Source: CAD feature listing. Evaluate the final solid. Frame: model axes, mm. Give positions to 0.01 mm unless a question says otherwise; leave off trailing zeros. Write each loop counter-clockwise with the first axis right and the second up, starting at its lowest first coordinate (ties: lowest second). Pieces come first, ordered by that corner, then holes. Notation, with made-up numbers: (23, -0.5) -> (47, -0.5) arc R34 ccw to (47, 33.5) -> close; hole circle Ø1 at (-11.5, 67). An arc over 180 degrees is marked (long way). Use a Markdown table: item, result. Add a question column.
```python
from build123d import *

# Parameters (mm, degrees)
BOSS_EXTRUDE1_DEPTH = 6
SKETCH2_R           = 12.45
BOSS_EXTRUDE2_DEPTH = 5.25
CUT_EXTRUDE2_REACH  = 13.25
SKETCH5_R           = 1.6
SKETCH6_R           = 2.75
CUT_EXTRUDE3_DEPTH  = 3.2
SKETCH7_R           = 2.75
CUT_EXTRUDE4_DEPTH  = 3.2
CUT_EXTRUDE7_REACH  = 8
SKETCH10_R          = 9.95
CUT_EXTRUDE8_REACH  = 13.25
SKETCH11_R          = 1.6
SKETCH12_R          = 2.75
CUT_EXTRUDE9_DEPTH  = 3
CUT_EXTRUDE10_DEPTH = 3
CUT_EXTRUDE11_REACH = 13.25
SKETCH14_R          = 1.6
SKETCH15_R          = 2.75
CUT_EXTRUDE12_DEPTH = 1.5
CUT_EXTRUDE13_REACH = 13.25
SKETCH16_R          = 1.1


with BuildPart() as part:
    # Sketch1 → Boss-Extrude1 (new body)
    with BuildSketch(Plane.XY):
        with BuildLine():
            Line((53.452478751, 19.630204959), (350.418509131, 15.138345609))
            ThreePointArc((350.418509131, 15.138345609), (370.113739503, -5.161848985), (349.813544909, -24.857079358))
            Line((349.813544909, -24.857079358), (52.847514529, -20.365220008))
            ThreePointArc((52.847514529, -20.365220008), (33.152284157, -0.065025413), (53.452478751, 19.630204959))
        make_face()
    extrude(amount=BOSS_EXTRUDE1_DEPTH)

    # Sketch2 → Boss-Extrude2 (add)
    with BuildSketch(Plane(origin=(0, 0, 0), x_dir=(-1, 0, 0), z_dir=(0, 0, -1))):
        with Locations((-53.14999664, -0.367507524)):
            Circle(SKETCH2_R)
    extrude(amount=BOSS_EXTRUDE2_DEPTH)

    # Sketch5 → Cut-Extrude2 (cut, up to next)
    with BuildSketch(Plane.XY.offset(6), mode=Mode.PRIVATE) as cut_extrude2_sk1:
        with Locations((80.82937417, 15.215648985)):
            Circle(SKETCH5_R)
    cut_extrude2_tool1 = extrude(cut_extrude2_sk1.sketch, amount=-CUT_EXTRUDE2_REACH, mode=Mode.PRIVATE) & part.part
    add(cut_extrude2_tool1.solids().sort_by_distance((80.829374, 15.215649, 6))[0], mode=Mode.SUBTRACT)
    # Sketch5 → Cut-Extrude2 (cut, up to next)
    with BuildSketch(Plane.XY.offset(6), mode=Mode.PRIVATE) as cut_extrude2_sk2:
        with Locations((46.471460884, -0.26648909)):
            Circle(SKETCH5_R)
    cut_extrude2_tool2 = extrude(cut_extrude2_sk2.sketch, amount=-CUT_EXTRUDE2_REACH, mode=Mode.PRIVATE) & part.part
    add(cut_extrude2_tool2.solids().sort_by_distance((46.471461, -0.266489, 6))[0], mode=Mode.SUBTRACT)
    # Sketch5 → Cut-Extrude2 (cut, up to next)
    with BuildSketch(Plane.XY.offset(6), mode=Mode.PRIVATE) as cut_extrude2_sk3:
        with Locations((80.345467382, -16.77642084)):
            Circle(SKETCH5_R)
    cut_extrude2_tool3 = extrude(cut_extrude2_sk3.sketch, amount=-CUT_EXTRUDE2_REACH, mode=Mode.PRIVATE) & part.part
    add(cut_extrude2_tool3.solids().sort_by_distance((80.345467, -16.776421, 6))[0], mode=Mode.SUBTRACT)

    # Sketch6 → Cut-Extrude3 (cut)
    with BuildSketch(Plane(origin=(0, 0, 0), x_dir=(-1, 0, 0), z_dir=(0, 0, -1))):
        with Locations((-80.345467382, -16.77642084)):
            Circle(SKETCH6_R)
        with Locations((-80.82937417, 15.215648985)):
            Circle(SKETCH6_R)
    extrude(amount=-CUT_EXTRUDE3_DEPTH, mode=Mode.SUBTRACT)

    # Sketch7 → Cut-Extrude4 (cut)
    with BuildSketch(Plane(origin=(0, 0, -5.25), x_dir=(-1, 0, 0), z_dir=(0, 0, -1))):
        with Locations((-46.471460884, -0.26648909)):
            Circle(SKETCH7_R)
    extrude(amount=-CUT_EXTRUDE4_DEPTH, mode=Mode.SUBTRACT)

    # Sketch10 → Cut-Extrude7 (cut, up to next)
    with BuildSketch(Plane(origin=(0, 0, 0), x_dir=(-1, 0, 0), z_dir=(0, 0, -1)), mode=Mode.PRIVATE) as cut_extrude7_sk1:
        with Locations((-350.11602702, -4.859366874)):
            Circle(SKETCH10_R)
    cut_extrude7_tool1 = extrude(cut_extrude7_sk1.sketch, amount=-CUT_EXTRUDE7_REACH, mode=Mode.PRIVATE) & part.part
    add(cut_extrude7_tool1.solids().sort_by_distance((350.116027, -4.859367, 0))[0], mode=Mode.SUBTRACT)

    # Sketch11 → Cut-Extrude8 (cut, up to next)
    with BuildSketch(Plane.XY.offset(6), mode=Mode.PRIVATE) as cut_extrude8_sk1:
        with Locations((207.693855596, 5.295802586)):
            Circle(SKETCH11_R)
    cut_extrude8_tool1 = extrude(cut_extrude8_sk1.sketch, amount=-CUT_EXTRUDE8_REACH, mode=Mode.PRIVATE) & part.part
    add(cut_extrude8_tool1.solids().sort_by_distance((207.693856, 5.295803, 6))[0], mode=Mode.SUBTRACT)
    # Sketch11 → Cut-Extrude8 (cut, up to next)
    with BuildSketch(Plane.XY.offset(6), mode=Mode.PRIVATE) as cut_extrude8_sk2:
        with Locations((207.451869907, -10.702367401)):
            Circle(SKETCH11_R)
    cut_extrude8_tool2 = extrude(cut_extrude8_sk2.sketch, amount=-CUT_EXTRUDE8_REACH, mode=Mode.PRIVATE) & part.part
    add(cut_extrude8_tool2.solids().sort_by_distance((207.45187, -10.702367, 6))[0], mode=Mode.SUBTRACT)
    # Sketch11 → Cut-Extrude8 (cut, up to next)
    with BuildSketch(Plane.XY.offset(6), mode=Mode.PRIVATE) as cut_extrude8_sk3:
        with Locations((168.025770935, 5.895815512)):
            Circle(SKETCH11_R)
    cut_extrude8_tool3 = extrude(cut_extrude8_sk3.sketch, amount=-CUT_EXTRUDE8_REACH, mode=Mode.PRIVATE) & part.part
    add(cut_extrude8_tool3.solids().sort_by_distance((168.025771, 5.895816, 6))[0], mode=Mode.SUBTRACT)
    # Sketch11 → Cut-Extrude8 (cut, up to next)
    with BuildSketch(Plane.XY.offset(6), mode=Mode.PRIVATE) as cut_extrude8_sk4:
        with Locations((167.783785246, -10.102354474)):
            Circle(SKETCH11_R)
    cut_extrude8_tool4 = extrude(cut_extrude8_sk4.sketch, amount=-CUT_EXTRUDE8_REACH, mode=Mode.PRIVATE) & part.part
    add(cut_extrude8_tool4.solids().sort_by_distance((167.783785, -10.102354, 6))[0], mode=Mode.SUBTRACT)

    # Sketch12 → Cut-Extrude9 (cut)
    with BuildSketch(Plane(origin=(0, 0, 0), x_dir=(-1, 0, 0), z_dir=(0, 0, -1))):
        with Locations((-207.451869907, -10.702367401)):
            Circle(SKETCH12_R)
        with Locations((-207.693855596, 5.295802586)):
            Circle(SKETCH12_R)
        with Locations((-168.025770935, 5.895815512)):
            Circle(SKETCH12_R)
        with Locations((-167.783785246, -10.102354474)):
            Circle(SKETCH12_R)
    extrude(amount=-CUT_EXTRUDE9_DEPTH, mode=Mode.SUBTRACT)

    # Sketch13 → Cut-Extrude10 (cut)
    with BuildSketch(Plane.XY.offset(6)):
        Polygon((289.732546516, 16.056271502), (289.422502353, -4.441383793), (320.418956702, -4.910231066), (320.729000866, 15.58742423), align=None)
    extrude(amount=-CUT_EXTRUDE10_DEPTH, mode=Mode.SUBTRACT)

    # Sketch14 → Cut-Extrude11 (cut, up to next)
    with BuildSketch(Plane.XY.offset(6), mode=Mode.PRIVATE) as cut_extrude11_sk1:
        with Locations((312.048483794, 3.717351637)):
            Circle(SKETCH14_R)
    cut_extrude11_tool1 = extrude(cut_extrude11_sk1.sketch, amount=-CUT_EXTRUDE11_REACH, mode=Mode.PRIVATE) & part.part
    add(cut_extrude11_tool1.solids().sort_by_distance((312.048484, 3.717352, 6))[0], mode=Mode.SUBTRACT)
    # Sketch14 → Cut-Extrude11 (cut, up to next)
    with BuildSketch(Plane.XY.offset(6), mode=Mode.PRIVATE) as cut_extrude11_sk2:
        with Locations((298.050085055, 3.929089115)):
            Circle(SKETCH14_R)
    cut_extrude11_tool2 = extrude(cut_extrude11_sk2.sketch, amount=-CUT_EXTRUDE11_REACH, mode=Mode.PRIVATE) & part.part
    add(cut_extrude11_tool2.solids().sort_by_distance((298.050085, 3.929089, 6))[0], mode=Mode.SUBTRACT)

    # Sketch15 → Cut-Extrude12 (cut)
    with BuildSketch(Plane(origin=(0, 0, 0), x_dir=(-1, 0, 0), z_dir=(0, 0, -1))):
        with Locations((-298.050085055, 3.929089115)):
            Circle(SKETCH15_R)
        with Locations((-312.048483794, 3.717351637)):
            Circle(SKETCH15_R)
    extrude(amount=-CUT_EXTRUDE12_DEPTH, mode=Mode.SUBTRACT)

    # Sketch16 → Cut-Extrude13 (cut, up to next)
    with BuildSketch(Plane.XY.offset(6), mode=Mode.PRIVATE) as cut_extrude13_sk1:
        with Locations((92.548117071, 17.038621984)):
            Circle(SKETCH16_R)
    cut_extrude13_tool1 = extrude(cut_extrude13_sk1.sketch, amount=-CUT_EXTRUDE13_REACH, mode=Mode.PRIVATE) & part.part
    add(cut_extrude13_tool1.solids().sort_by_distance((92.548117, 17.038622, 6))[0], mode=Mode.SUBTRACT)
    # Sketch16 → Cut-Extrude13 (cut, up to next)
    with BuildSketch(Plane.XY.offset(6), mode=Mode.PRIVATE) as cut_extrude13_sk2:
        with Locations((92.003649271, -18.957260486)):
            Circle(SKETCH16_R)
    cut_extrude13_tool2 = extrude(cut_extrude13_sk2.sketch, amount=-CUT_EXTRUDE13_REACH, mode=Mode.PRIVATE) & part.part
    add(cut_extrude13_tool2.solids().sort_by_distance((92.003649, -18.95726, 6))[0], mode=Mode.SUBTRACT)
    # Sketch16 → Cut-Extrude13 (cut, up to next)
    with BuildSketch(Plane.XY.offset(6), mode=Mode.PRIVATE) as cut_extrude13_sk3:
        with Locations((151.905473082, 16.140792376)):
            Circle(SKETCH16_R)
    cut_extrude13_tool3 = extrude(cut_extrude13_sk3.sketch, amount=-CUT_EXTRUDE13_REACH, mode=Mode.PRIVATE) & part.part
    add(cut_extrude13_tool3.solids().sort_by_distance((151.905473, 16.140792, 6))[0], mode=Mode.SUBTRACT)
    # Sketch16 → Cut-Extrude13 (cut, up to next)
    with BuildSketch(Plane.XY.offset(6), mode=Mode.PRIVATE) as cut_extrude13_sk4:
        with Locations((151.361005282, -19.855090094)):
            Circle(SKETCH16_R)
    cut_extrude13_tool4 = extrude(cut_extrude13_sk4.sketch, amount=-CUT_EXTRUDE13_REACH, mode=Mode.PRIVATE) & part.part
    add(cut_extrude13_tool4.solids().sort_by_distance((151.361005, -19.85509, 6))[0], mode=Mode.SUBTRACT)
    # Sketch16 → Cut-Extrude13 (cut, up to next)
    with BuildSketch(Plane.XY.offset(6), mode=Mode.PRIVATE) as cut_extrude13_sk5:
        with Locations((222.744414799, 15.069294191)):
            Circle(SKETCH16_R)
    cut_extrude13_tool5 = extrude(cut_extrude13_sk5.sketch, amount=-CUT_EXTRUDE13_REACH, mode=Mode.PRIVATE) & part.part
    add(cut_extrude13_tool5.solids().sort_by_distance((222.744415, 15.069294, 6))[0], mode=Mode.SUBTRACT)
    # Sketch16 → Cut-Extrude13 (cut, up to next)
    with BuildSketch(Plane.XY.offset(6), mode=Mode.PRIVATE) as cut_extrude13_sk6:
        with Locations((283.996308166, 14.142808123)):
            Circle(SKETCH16_R)
    cut_extrude13_tool6 = extrude(cut_extrude13_sk6.sketch, amount=-CUT_EXTRUDE13_REACH, mode=Mode.PRIVATE) & part.part
    add(cut_extrude13_tool6.solids().sort_by_distance((283.996308, 14.142808, 6))[0], mode=Mode.SUBTRACT)


solid = part.part
```
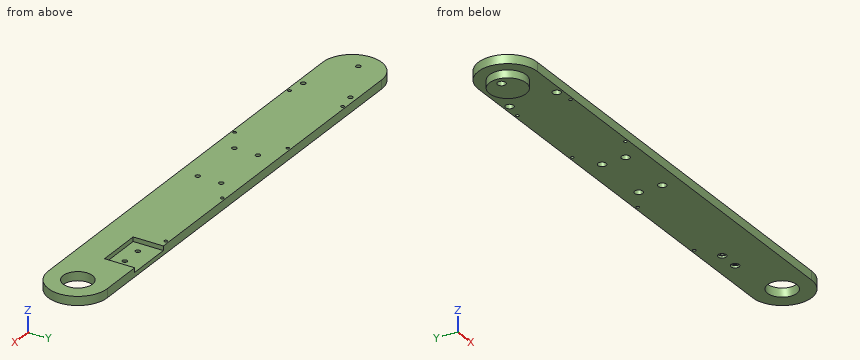
(1) First-contact query: pin 1 Ø6 at (x, y) = (208.5, -11.5) entering from -Z; pin 2 Ø5 at (y, z) = (-8.5, -1) entering from -X; pin 3 Ø3.5 at (x, y) = (207.45, -10.7) entering from -Z; pin 4 Ø7 at (x, y) = (80.83, 15.22) entering from +Z. Flat tips, straight axial feed; report the tip coordinate or a pass-through.
(2) Material intervals for L1, parallel to Y at x = 151.5, z = 3; L2, parallel to X at y = -1.5, z = 1.5; L3, parallel to Z at x = 261, y = 2.5, sorted ascending.
(3) Cut plane A-A on x = 330. Return the cut outline in (y, z), then the cut area to 3 significant figures.
Output:
| question | item | result |
|---|---|---|
| 1 | pin 1 | z = 0 |
| 1 | pin 2 | x = 34.02 |
| 1 | pin 3 | z = 3 |
| 1 | pin 4 | z = 6 |
| 2 | L1 | -21.86 to -20.95, -18.76 to 15.12, 17.16 to 18.15 |
| 2 | L2 | 33.18 to 45.45, 47.49 to 340.75, 359.48 to 369.83 |
| 2 | L3 | 0 to 6 |
| 3 | outline | (-24.56, 0) -> (15.45, 0) -> (15.45, 6) -> (-24.56, 6) -> close |
| 3 | area | 240 mm^2 |
